For this review, take the finished solid that the model builds, in its own axes (mm). A direction names the side the tool comes from. Coordinates: 2 decimals unless noted, no trailing zeros. Order: outer loops, then holes, each group sorted by start corner. A loop starts at its lowest first (then second) coordinate and runs counter-clockwise, first axis right, second up. Notation, with made-up numbers: (19.5, 81.5) - (35.5, 81.5) arc R22 ccw to (35.5, 115.5) - close; hole circle Ø8 at (61, -1.5). An arc over 180 degrees is marked (long way). One line per item, written item: value. Start each with the question number.
(1) Mouldability with a two-part tool opening along Y and no side actions: class faces 1 (the flat face through (13.5, 23, 1)), 2 (the flat face through (17, 24.5, 1)), 3 (the flat face through (-8, 32, 1)) as released by +Y, released by -Y, zero draft, split by the parting line, or undercut.
(2) For faces 4 (the flat face through (-4, 54, 1)), 5 (the flat face through (1.9, 48.4, 1.5)), 6 (the flat face through (4.5, -8, 1)), list the 3-axis set-ups (+Z, -Z, +X, -X, +Y, -Y) from which the entire face can be reached by the end or side of a thin tool; tool diameter is ignored.
(3) Consider section C-C on y = 30. Write out the cut boundary in (x, z).
(4) Consider section B-B on z = 2.3. Count the separate pieces of the cut face and the enclosed holes in it, then the cut area to 3 significant figures.
(5) Clearance check with flat-ended pins moving along their axes: pin 1 (1.5 mm diameter, centred on x = 18, z = 1, fed in from +Y); pin 2 (1.5 mm diameter, centred on x = 7, z = 1, fed in from +Y); pin 3 (12 mm diameter, centred on x = 11, y = 14, fed in from -Z); pin 4 (0.9 mm diameter, centred on y = 28.5, z = 1.5, fed in from +X). State where each tip first meets the part, or that it passes through.
(6) Consider section A-A on y = 40.5. Write out the cut boundary in (x, z).
(7) To check wall thickness, follow line 1 along Y through (x, z) = (11, 1.9); line 2 along Y through (x, z) = (4, 2.45); line 3 along Y through (x, z) = (3, 1.65). State the ranges of each line that lie inside material, in increasing order.
```python
from build123d import *

# Parameters (mm, degrees)
SKETCH_1_R                   = 1.55
SKETCH_1_R_2                 = 1.3
EXTRUDE_1_DEPTH              = 3
SKETCH_3_R                   = 1.55
CUT_EXTRUDE_1_DEPTH          = 59.017238817
HOLE_WIZARD_M3_1_D           = 3.1
HOLE_WIZARD_M3_1_CSINK_D     = 6
HOLE_WIZARD_M3_1_CSINK_ANGLE = 90
FILLET_1_R                   = 1


with BuildPart() as part:
    # 草图1 → 凸台-拉伸1 (new body)
    with BuildSketch(Plane.XY):
        Polygon((-19.35, -7), (-4.509137286, -21), (-4.509137286, -24.5), (8.5, -24.5), (8.5, -21), (13.5, -21), (13.5, -24.5), (21, -24.5), (21, -12.5), (21, -5.443486713), (21, 5.443486713), (21, 12.5), (21, 24.5), (13.5, 24.5), (13.5, 21), (8.5, 21), (8.5, 24.5), (0, 36.639258057), (0, 46.5), (3.5, 50), (3.5, 50.5), (2.5, 50.5), (2.5, 53), (3.5, 53), (3.5, 54), (-11.5, 54), (-11.5, 53), (-10.5, 53), (-10.5, 50.5), (-11.5, 50.5), (-11.5, 50), (-8, 46.5), (-8, 17.70692473), (-10.85, 15.01840178), (-19.35, 7), (-19.35, 5.629370629), align=None)
        with Locations((-16.5, 4)):
            Circle(SKETCH_1_R, mode=Mode.SUBTRACT)
        with Locations((-16.5, -4)):
            Circle(SKETCH_1_R, mode=Mode.SUBTRACT)
        with Locations((16.5, 4)):
            Circle(SKETCH_1_R, mode=Mode.SUBTRACT)
        with Locations((16.5, -4)):
            Circle(SKETCH_1_R, mode=Mode.SUBTRACT)
        with Locations((0, 18)):
            Circle(SKETCH_1_R_2, mode=Mode.SUBTRACT)
        with Locations(Location((0, -18, 0), (0, 0, 180))):
            Circle(SKETCH_1_R_2, mode=Mode.SUBTRACT)
        with Locations((-4, 40.5)):
            Circle(SKETCH_1_R, mode=Mode.SUBTRACT)
        with Locations((-4, 32.5)):
            Circle(SKETCH_1_R, mode=Mode.SUBTRACT)
        Polygon((0, 24.5), (4.837676234, 24.5), (0, 31.40891767), align=None, mode=Mode.SUBTRACT)
        Polygon((-4.245815128, 13), (4.5, 13), (4.5, 3), (-10.5, 3), (-10.5, 7.100168575), align=None, mode=Mode.SUBTRACT)
        Polygon((-10.5, -3), (-10.5, -7.100168575), (-4.245815128, -13), (4.5, -13), (4.5, -3), align=None, mode=Mode.SUBTRACT)
    extrude(amount=EXTRUDE_1_DEPTH)

    # 草图3 → 切除-拉伸1 (cut, through all)
    with BuildSketch(Plane.XY.offset(3)):
        with Locations((11, 5)):
            Circle(SKETCH_3_R)
        with Locations((7, 5)):
            Circle(SKETCH_3_R)
        with Locations((11, -5)):
            Circle(SKETCH_3_R)
        with Locations((7, -5)):
            Circle(SKETCH_3_R)
    extrude(amount=-CUT_EXTRUDE_1_DEPTH, mode=Mode.SUBTRACT)

    # M3 六角凹锥坑螺钉的锥形沉头孔1 (through all)
    with Locations(Plane(origin=(16.5, -4, 3), x_dir=(1, 0, 0), z_dir=(0, 0, 1))):
        with Locations((0, 0), (0, 8)):
            CounterSinkHole(HOLE_WIZARD_M3_1_D / 2, HOLE_WIZARD_M3_1_CSINK_D / 2, counter_sink_angle=HOLE_WIZARD_M3_1_CSINK_ANGLE)

    # 圆角1
    # the kernel refuses this fillet: 1 mm, written as the material it adds along each edge
    with BuildSketch(Plane(origin=(8.5, 21, 0), x_dir=(0, 1, 0), z_dir=(0, 0, 1)), Plane(origin=(13.5, 21, 0), x_dir=(-1, 0, 0), z_dir=(0, 0, 1)), Plane(origin=(13.5, -21, 0), x_dir=(0, -1, 0), z_dir=(0, 0, 1)), Plane(origin=(8.5, -21, 0), x_dir=(1, 0, 0), z_dir=(0, 0, 1)), Plane(origin=(4.5, -13, 0), x_dir=(-1, 0, 0), z_dir=(0, 0, 1)), Plane(origin=(4.5, -3, 0), x_dir=(0, -1, 0), z_dir=(0, 0, 1)), Plane(origin=(-10.5, 3, 0), x_dir=(0, 1, 0), z_dir=(0, 0, 1)), Plane(origin=(4.5, 3, 0), x_dir=(-1, 0, 0), z_dir=(0, 0, 1)), Plane(origin=(4.5, 13, 0), x_dir=(0, -1, 0), z_dir=(0, 0, 1))) as fillet_1_piece_1:
        with BuildLine():
            CenterArc((FILLET_1_R, -FILLET_1_R), FILLET_1_R, 90, 90)
            Line((0, -FILLET_1_R), (0, 0))
            Line((0, 0), (FILLET_1_R, 0))
        make_face()
    extrude(amount=3)
    with BuildSketch(Plane(origin=(-4.509137286, -21, 0), x_dir=(-0.7274135642622264, 0.686199319824294, 0), z_dir=(0, 0, 1))) as fillet_1_piece_2:
        with BuildLine():
            CenterArc((FILLET_1_R * 0.431392395733, FILLET_1_R), FILLET_1_R, 223.33, 46.67)
            Line((-FILLET_1_R * 0.296021168529, FILLET_1_R * 0.313800680176), (0, 0))
            Line((0, 0), (FILLET_1_R * 0.431392395733, 0))
        make_face()
    extrude(amount=3)
    with BuildSketch(Plane(origin=(-10.5, -7.100168575, 0), x_dir=(0, 1, 0), z_dir=(0, 0, 1)), Plane(origin=(-10.5, 7.100168575, 0), x_dir=(0.7274135642622253, 0.6861993198242954, 0), z_dir=(0, 0, 1)), Plane(origin=(-8, 17.70692473, 0), x_dir=(-0.7274135642622253, -0.6861993198242954, 0), z_dir=(0, 0, 1))) as fillet_1_piece_3:
        with BuildLine():
            CenterArc((FILLET_1_R * 0.431392395733, -FILLET_1_R), FILLET_1_R, 90, 46.67)
            Line((-FILLET_1_R * 0.296021168529, -FILLET_1_R * 0.313800680176), (0, 0))
            Line((0, 0), (FILLET_1_R * 0.431392395733, 0))
        make_face()
    extrude(amount=3)
    with BuildSketch(Plane(origin=(-4.245815128, -13, 0), x_dir=(-0.727413564262223, 0.6861993198242976, 0), z_dir=(0, 0, 1))) as fillet_1_piece_4:
        with BuildLine():
            CenterArc((FILLET_1_R * 0.397240900512, -FILLET_1_R), FILLET_1_R, 90, 43.33)
            Line((-FILLET_1_R * 0.288958419312, -FILLET_1_R * 0.272586435738), (0, 0))
            Line((0, 0), (FILLET_1_R * 0.397240900512, 0))
        make_face()
    extrude(amount=3)
    with BuildSketch(Plane(origin=(-10.5, -3, 0), x_dir=(0, -1, 0), z_dir=(0, 0, 1))) as fillet_1_piece_5:
        with BuildLine():
            CenterArc((FILLET_1_R, FILLET_1_R), FILLET_1_R, 180, 90)
            Line((0, FILLET_1_R), (0, 0))
            Line((0, 0), (FILLET_1_R, 0))
        make_face()
    extrude(amount=3)
    with BuildSketch(Plane(origin=(-4.245815128, 13, 0), x_dir=(-0.727413564262223, -0.6861993198242976, 0), z_dir=(0, 0, 1))) as fillet_1_piece_6:
        with BuildLine():
            CenterArc((FILLET_1_R * 0.397240900512, FILLET_1_R), FILLET_1_R, 226.67, 43.33)
            Line((-FILLET_1_R * 0.288958419312, FILLET_1_R * 0.272586435738), (0, 0))
            Line((0, 0), (FILLET_1_R * 0.397240900512, 0))
        make_face()
    extrude(amount=3)
    with BuildSketch(Plane(origin=(-8, 46.5, 0), x_dir=(0, -1, 0), z_dir=(0, 0, 1)), Plane(origin=(0, 46.5, 0), x_dir=(0.7071067811865551, 0.70710678118654, 0), z_dir=(0, 0, 1))) as fillet_1_piece_7:
        with BuildLine():
            CenterArc((FILLET_1_R * 0.414213562373, -FILLET_1_R), FILLET_1_R, 90, 45)
            Line((-FILLET_1_R * 0.292893218813, -FILLET_1_R * 0.292893218813), (0, 0))
            Line((0, 0), (FILLET_1_R * 0.414213562373, 0))
        make_face()
    extrude(amount=3)
    with BuildSketch(Plane(origin=(0, 36.639258057, 0), x_dir=(0, 1, 0), z_dir=(0, 0, 1))) as fillet_1_piece_8:
        with BuildLine():
            CenterArc((FILLET_1_R * 0.315298788879, -FILLET_1_R), FILLET_1_R, 90, 35)
            Line((-FILLET_1_R * 0.258277647472, -FILLET_1_R * 0.180847955711), (0, 0))
            Line((0, 0), (FILLET_1_R * 0.315298788879, 0))
        make_face()
    extrude(amount=3)
    # the kernel refuses this fillet: 1 mm, written as the material it takes off along each edge
    with BuildSketch(Plane(origin=(13.5, 24.5, -2.5), x_dir=(1, 0, 0), z_dir=(0, 0, 1)), Plane(origin=(21, 24.5, -2.5), x_dir=(0, -1, 0), z_dir=(0, 0, 1)), Plane(origin=(21, -24.5, -2.5), x_dir=(-1, 0, 0), z_dir=(0, 0, 1)), Plane(origin=(13.5, -24.5, -2.5), x_dir=(0, 1, 0), z_dir=(0, 0, 1)), Plane(origin=(8.5, -24.5, -2.5), x_dir=(-1, 0, 0), z_dir=(0, 0, 1)), Plane(origin=(-4.509137286, -24.5, -2.5), x_dir=(0, 1, 0), z_dir=(0, 0, 1)), Plane(origin=(-11.5, 53, -2.5), x_dir=(0, 1, 0), z_dir=(0, 0, 1)), Plane(origin=(-11.5, 54, -2.5), x_dir=(1, 0, 0), z_dir=(0, 0, 1)), Plane(origin=(3.5, 54, -2.5), x_dir=(0, -1, 0), z_dir=(0, 0, 1)), Plane(origin=(3.5, 53, -2.5), x_dir=(-1, 0, 0), z_dir=(0, 0, 1))) as fillet_1_2_piece_1:
        with BuildLine():
            CenterArc((FILLET_1_R, -FILLET_1_R), FILLET_1_R, 90, 90)
            Line((0, -FILLET_1_R), (0, 0))
            Line((0, 0), (FILLET_1_R, 0))
        make_face()
    extrude(amount=8, mode=Mode.SUBTRACT)
    with BuildSketch(Plane(origin=(-19.35, -7, -1.078480989), x_dir=(0.7274135642622251, -0.6861993198242955, 0), z_dir=(0, 0, 1)), Plane(origin=(-19.35, 7, -1.078480989), x_dir=(0, -1, 0), z_dir=(0, 0, 1))) as fillet_1_2_piece_2:
        with BuildLine():
            CenterArc((FILLET_1_R * 0.431392395733, FILLET_1_R), FILLET_1_R, 223.33, 46.67)
            Line((-FILLET_1_R * 0.296021168529, FILLET_1_R * 0.313800680176), (0, 0))
            Line((0, 0), (FILLET_1_R * 0.431392395733, 0))
        make_face()
    extrude(amount=5.156961979, mode=Mode.SUBTRACT)
    with BuildSketch(Plane(origin=(-11.5, 50.5, -2.165063509), x_dir=(1, 0, 0), z_dir=(0, 0, 1))) as fillet_1_2_piece_3:
        with BuildLine():
            CenterArc((0.866025404, -1), FILLET_1_R, 90, 60)
            Line((0, -0.5), (0, 0))
            Line((0, 0), (0.866025404, 0))
        make_face()
    extrude(amount=7.330127019, mode=Mode.SUBTRACT)
    with BuildSketch(Plane(origin=(3.5, 50.5, -2.165063509), x_dir=(0, -1, 0), z_dir=(0, 0, 1))) as fillet_1_2_piece_4:
        with BuildLine():
            CenterArc((1, -0.866025404), FILLET_1_R, 120, 60)
            Line((0, -0.866025404), (0, 0))
            Line((0, 0), (0.5, 0))
        make_face()
    extrude(amount=7.330127019, mode=Mode.SUBTRACT)
    with BuildSketch(Plane(origin=(8.5, 24.5, -0.788246972), x_dir=(0, -1, 0), z_dir=(0, 0, 1))) as fillet_1_2_piece_5:
        with BuildLine():
            CenterArc((FILLET_1_R * 0.315298788879, -FILLET_1_R), FILLET_1_R, 90, 35)
            Line((-FILLET_1_R * 0.258277647472, -FILLET_1_R * 0.180847955711), (0, 0))
            Line((0, 0), (FILLET_1_R * 0.315298788879, 0))
        make_face()
    extrude(amount=4.576493944, mode=Mode.SUBTRACT)


solid = part.part
```
Geometry check:
1. face 1: zero draft
1. face 2: released by +Y
1. face 3: undercut
2. face 4: +Z, -Z, +X, -X, +Y
2. face 5: +Z, -Z, +X
2. face 6: +Z, -Z
3. outline: (-8, 0) - (0, 0) - (0, 3) - (-8, 3) - close; (0.99, 0) - (4.65, 0) - (4.65, 3) - (0.99, 3) - close
4. separate pieces: 1
4. enclosed holes: 15
4. area: 1,590 mm^2
5. pin 1: stops at y = 24.5
5. pin 2: stops at y = 27.71
5. pin 3: stops at z = 0
5. pin 4: stops at x = 6.01
6. outline: (-8, 0) - (-5.55, 0) - (-5.55, 3) - (-8, 3) - close; (-2.45, 0) - (0, 0) - (0, 3) - (-2.45, 3) - close
7. line 1: y = -21 to -6.55, -3.45 to 3.45, 6.55 to 21
7. line 2: y = -24.5 to -12.87, -3.13 to 3.13, 12.87 to 24.5, 25.7 to 30.93
7. line 3: y = -24.5 to -13, -3 to 3, 13 to 24.5, 27.12 to 32.35, 49.5 to 50.43, 53.13 to 53.87
